Part print with two shaded views. Sizes in mm from the minimum x, y, z corner. A direction names the side the tool comes from. Coordinates: 2 decimals unless noted, no trailing zeros. Loops run counter-clockwise (first coordinate to the right, second up) from the corner with the lowest first, then second, coordinate; pieces in that order, holes last. Notation, with made-up numbers: (-29.75, -30) -> (10.25, -30) arc R21 cw to (10.25, 8) -> close; hole circle Ø10 at (27.5, -29). An arc over 180 degrees is marked (long way). Write each question's results on one line, items separated by ' | '.
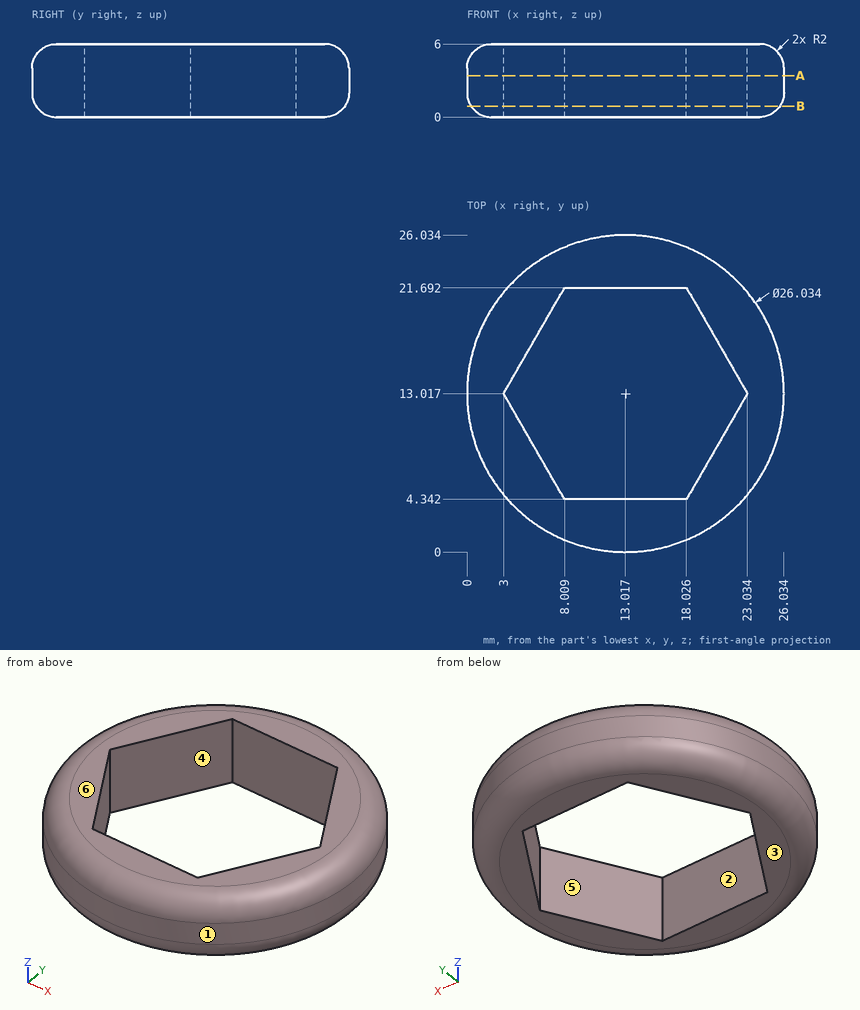
Q1. Cut at A-A on z = 3.4. Write the cut outline in (x, y) (1 decimal).
Results are:
outline: circle Ø26 at (13, 13); hole (3, 13) -> (8, 4.3) -> (18, 4.3) -> (23, 13) -> (18, 21.7) -> (8, 21.7) -> close
Q2. Pull direction Y, two halves, no side cores. Call the marked faces 1, 2, 3 and 4: +Y half, -Y half, draft (parallel to the pull), parting line (faces both ways), or undercut.
Results are:
face 1: parting line | face 2: undercut | face 3: draft | face 4: undercut
Q3. Which spindle directions (+Z, -Z, +X, -X, +Y, -Y) get a long thin tool onto all of the face, cutting with end or side? Do the marked faces 5 and 6. Say none if no direction does.
Results are:
face 5: +Z, -Z | face 6: +Z, +X, -X, +Y, -Y
Q4. Drop flat-ended pins along their axis: pin 1 (3 mm diameter, centred on x = 8.5, z = 4.5, fed in from +Y) (1 decimal); pin 2 (1.5 mm diameter, centred on y = 18.5, z = 2, fed in from +X). Give the stop position or say it passes through.
Results are:
pin 1: y = 25.7 | pin 2: x = 25.14
Q5. Cut at B-B on z = 0.9. Write the cut outline in (x, y) (1 decimal), and give its area (3 significant figures).
Results are:
outline: circle Ø25.4 at (13, 13); hole (3, 13) -> (8, 4.3) -> (18, 4.3) -> (23, 13) -> (18, 21.7) -> (8, 21.7) -> close | area: 245 mm^2
Q6. Wall check: L1, parallel to X at y = 17, z = 3.2 (1 decimal); L2, parallel to X at y = 6.75, z = 2.75 (1 decimal); L3, parallel to Y at x = 12.5, z = 0.85 (1 decimal). Give the ranges that are in metal, low to high. Write a range as from..to.
Results are:
L1: 0.6..5.3, 20.7..25.4 | L2: 1.6..6.6, 19.4..24.4 | L3: 0.4..4.3, 21.7..25.7
